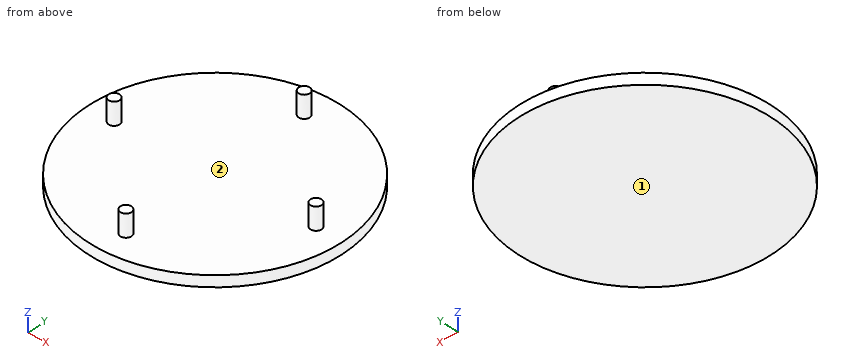
from build123d import *

# Parameters (mm, degrees)
SKETCH1_R           = 11.5
BOSS_EXTRUDE1_DEPTH = 1
SKETCH4_R           = 0.5
BOSS_EXTRUDE4_DEPTH = 2
CIRPATTERN3_COUNT   = 4


with BuildPart() as part:
    # Sketch1 → Boss-Extrude1 (new body)
    with BuildSketch(Plane.XY):
        with Locations((0, -0.253320711)):
            Circle(SKETCH1_R)
    extrude(amount=-BOSS_EXTRUDE1_DEPTH)

    # Sketch4 → Boss-Extrude4 (add)
    with BuildSketch(Plane.XY):
        with Locations((8.999235852, -0.117277767)):
            Circle(SKETCH4_R)
    boss_extrude4 = extrude(amount=BOSS_EXTRUDE4_DEPTH)

    # CirPattern3: Boss-Extrude4 ×4 about axis
    cirpattern3_axis = Axis((0, -0.253320711, 0), (0, 0, 1))
    for i in range(1, CIRPATTERN3_COUNT):
        add(boss_extrude4.rotate(cirpattern3_axis, i * 360 / CIRPATTERN3_COUNT))


solid = part.part
Geometry: final body of the model. Coordinates: model frame, mm. Face numbers are marked on the shaded views. A direction names the side the tool comes from. Coordinates: 2 decimals unless noted, no trailing zeros. Order: outer loops, then holes, each group sorted by start corner. A loop starts at its lowest first (then second) coordinate and runs counter-clockwise, first axis right, second up. Notation, with made-up numbers: M -33.5,34.5 L -9.5,34.5 A21 ccw -9.5,70.5 Z; hole C -39,14.25 d7. An arc over 180 degrees is marked long. One line per question, with ' | ' between items. Start each with the question number.
Item 1: Cut plane C-C, the plane x = 5.25. Return the cut outline in (y, z).
Item 2: Cut plane B-B, the plane y = -8. Return the cut outline in (x, z).
Item 3: Cut plane D-D, the plane z = -0.3. Return the cut outline in (x, y).
Item 4: Set-up query: the marked faces 1 and 2. Return all of +Z, -Z, +X, -X, +Y, -Y with unobstructed straight access to the full face (end or side cutting, diameter ignored); none if empty.
Item 5: Cut plane A-A, the plane z = 1.1. Return the cut outline in (x, y), then the cut area to 3 significant figures.
Item 6: Pin query (flat end, axial travel): pin 1 Ø1 at (x, z) = (-6, 1.5) entering from +Y; pin 2 Ø8 at (x, y) = (-8, 6.5) entering from +Z; pin 3 Ø11.5 at (x, y) = (4.5, 5) entering from +Z. Return the tip coordinate at first contact, or that it passes through.
Item 7: Ray query, probe 1 along Z at (x, y) = (-2.25, -3.5); probe 2 along Y at (x, z) = (0.25, -0.25); probe 3 along X at (y, z) = (-1, -0.75). Return the intervals inside material, ascending. Write a range as [from, to].
A:
1) outline: M -10.49,-1 L 9.98,-1 L 9.98,0 L -10.49,0 Z
2) outline: M -8.5,-1 L 8.5,-1 L 8.5,0 L -8.5,0 Z
3) outline: C 0,-0.25 d23
4) face 1: -Z, +X, -X, +Y, -Y | face 2: +Z
5) outline: C -9,-0.39 d1; C -0.14,8.75 d1; C 0.14,-9.25 d1; C 9,-0.12 d1 | area: 3.14 mm2
6) pin 1: passes through | pin 2: stops at z = 0 | pin 3: stops at z = 2
7) probe 1: z = [-1, 0] | probe 2: y = [-11.75, 11.24] | probe 3: x = [-11.48, 11.48]
